Solid Edge part; units mm, degrees
sketch "Sketch1" plane through (0, 0, 0) normal (0, -1, 0) x (1, 0, 0)
  line L0 (-25, 14.3343) -> (-25, -47.4657)
  line L1 (-25, -47.4657) -> (25, -47.4657)
  line L2 (25, -47.4657) -> (25, 14.3343)
  line L3 (25, 14.3343) -> (-25, 14.3343)
  dimension "D1" = 25
  dimension "D2" = 25
extrude "Protrusion1" add sketch "Sketch1" along normal blind 3
sketch "Sketch2" plane through (0, 0, 0) normal (0, -1, 0) x (1, 0, 0)
  line L0 (0, -1.4657) -> (-25, -1.4657)
  line L1 (-25, -1.4657) -> (-25, -47.4657)
  line L2 (-25, -47.4657) -> (25, -47.4657)
  line L3 (25, -47.4657) -> (25, -1.4657)
  line L4 (25, -1.4657) -> (0, -1.4657)
extrude "ExtrudedProtrusion_2" add sketch "Sketch2" along normal blind 52
sketch "Sketch3" plane through (25, -26, -16.5657) normal (1, 0, 0) x (0, 1, 0)
  line L0 (-21, -19.9) -> (9, -19.9)
  line L1 (9, -19.9) -> (9, 10.1)
  line L2 (9, 10.1) -> (-21, 10.1)
  line L3 (-21, 10.1) -> (-21, -19.9)
  dimension "D1" = 21
  dimension "D2" = 21
  dimension "D3" = 9
extrude "ExtrudedProtrusion_3" add sketch "Sketch3" along normal blind 13
sketch "Sketch4" plane through (-25, -26, -16.5657) normal (-1, 0, 0) x (0, 1, 0)
  circle A0 centre (0.7428, 8.2455) radius 2.5
extrude "ExtrudedProtrusion_4" add sketch "Sketch4" along normal blind 10
sketch "Sketch5" plane through (0, 0, -16.5657) normal (0, 1, 0) x (-1, 0, 0)
  circle A0 centre (22.5, 12.9) radius 1.5
  circle A1 centre (-22.5, -12.1) radius 1.5
  circle A2 centre (22.5, -12.1) radius 1.5
  circle A3 centre (-22.5, 12.9) radius 1.5
extrude "ExtrudedCutout_1" cut sketch "Sketch5" against normal blind 10
sketch "Sketch6" plane through (0, -26, -47.4657) normal (0, 0, -1) x (-1, 0, 0)
  circle A0 centre (-19, 7) radius 2.5
  dimension "D1" = 19
  dimension "D2" = 19
extrude "ExtrudedProtrusion_5" add sketch "Sketch6" along normal blind 8
sketch "Sketch7" plane through (19, -19, -55.4657) normal (0, 0, -1) x (-1, 0, 0)
  line L0 (-6, 5.8881) -> (-6, -7)
  line L1 (-6, -7) -> (7.7613, -7)
  line L2 (7.7613, -7) -> (7.7613, 5.8881)
  line L3 (7.7613, 5.8881) -> (-6, 5.8881)
  dimension "D1" = 6
extrude "ExtrudedProtrusion_6" add sketch "Sketch7" against normal blind 6
sketch "Sketch8" plane through (18.1194, -19.5559, -55.4657) normal (0, 0, -1) x (-1, 0, 0)
  circle A0 centre (-0.8806, 0.5559) radius 2.5
extrude "ExtrudedProtrusion_7" add sketch "Sketch8" along normal blind 6
Geometry: final body of the model. Coordinates: model frame, mm. A direction names the side the tool comes from. Round coordinates to 2 decimals unless told otherwise and drop trailing zeros. Order: outer loops, then holes, each group sorted by start corner. A loop starts at its lowest first (then second) coordinate and runs counter-clockwise, first axis right, second up.
Q1. Section B-B, the plane x = -22.5. Output: boundary loops of the cut face in (y, z).
Result sheet:
outline: (-52, -47.47) - (0, -47.47) - (0, -30.17) - (-10, -30.17) - (-10, -27.17) - (0, -27.17) - (0, -5.17) - (-10, -5.17) - (-10, -2.17) - (0, -2.17) - (0, 14.33) - (-3, 14.33) - (-3, -1.47) - (-52, -1.47) - close
Q2. Section D-D, the plane y = -4. Output: boundary loops of the cut face in (x, z).
Result sheet:
outline: (-25, -47.47) - (25, -47.47) - (25, -1.47) - (-25, -1.47) - close; hole circle Ø3 at (-22.5, -28.67); hole circle Ø3 at (-22.5, -3.67); hole circle Ø3 at (22.5, -28.67); hole circle Ø3 at (22.5, -3.67)
Q3. Section A-A, the plane x = 15. Output: boundary loops of the cut face in (y, z), and give its area (3 significant figures).
Result sheet:
outline: (-52, -47.47) - (0, -47.47) - (0, 14.33) - (-3, 14.33) - (-3, -1.47) - (-52, -1.47) - close; (-26, -55.47) - (-13.11, -55.47) - (-13.11, -49.47) - (-26, -49.47) - close
area: 2,520 mm2
Q4. Section C-C, the plane y = -46. Output: boundary loops of the cut face in (x, z), and give its area (3 significant figures).
Result sheet:
outline: (-25, -47.47) - (25, -47.47) - (25, -36.47) - (38, -36.47) - (38, -6.47) - (25, -6.47) - (25, -1.47) - (-25, -1.47) - close
area: 2,690 mm2
Q5. Pin query (flat end, axial travel): pin 1 (6.5 mm diameter, centred on y = -17, z = -51.5, fed in from +X); pin 2 (10 mm diameter, centred on y = -17.5, z = -8.5, fed in from -X); pin 3 (14.5 mm diameter, centred on x = 7, y = -39.5, fed in from +Z). Return the tip coordinate at first contact, or that it passes through.
Result sheet:
pin 1: stops at x = 25
pin 2: stops at x = -25
pin 3: stops at z = -1.47
Q6. Mould query, pull axis X, two halves, no side actions, for faces 6 (the face through (23, -10, -4)), 7 (the face through (20.84, -20.69, -58.42)), 8 (the face through (-29.93, -24.104, -27.029)). Classes: released by +X, released by -X, zero draft, split by the parting line, or undercut.
Result sheet:
face 6: undercut
face 7: split by the parting line
face 8: zero draft
Q7. Material intervals for probe 1 along Z at (x, y) = (-22.5, -5); probe 2 along Z at (x, y) = (22, -6); probe 3 along X at (y, z) = (-34, -46.5), sorted ascending.
Result sheet:
probe 1: z = -47.47 to -30.17, -27.17 to -5.17, -2.17 to -1.47
probe 2: z = -47.47 to -30.08, -27.25 to -5.08, -2.25 to -1.47
probe 3: x = -25 to 25
Q8. Access query for faces 1 (the face through (11.239, -20, -53)), 2 (the face through (23, -10, -29)), 3 (the face through (31, -32, -6.466)), 4 (the face through (17, -21, -49.466)), 5 (the face through (17, -21, -55.466)). Directions: +Z, -Z, +X, -X, +Y, -Y. A direction counts if a zero-diameter tool reaches every point of the face in a straight line with its end or side. Return the directions, or none.
Result sheet:
face 1: -Z, -X, +Y, -Y
face 2: +Y
face 3: +Z, +X, +Y, -Y
face 4: none
face 5: -Z
